The figure shows three views and two pictorial views of one solid part (mm, origin at its lowest corner). Answer the questions. Round coordinates to 2 decimals unless told otherwise and drop trailing zeros. Order: outer loops, then holes, each group sorted by start corner. A loop starts at its lowest first (then second) coordinate and runs counter-clockwise, first axis right, second up. Notation, with made-up numbers: (17, 16.25) -> (45, 16.25) arc R29 cw to (45, 39.25) -> close; hole circle Ø2 at (87, 72.25). An arc over 180 degrees is marked (long way). Return JSON: item names as keys, results as strings. Group by question number.
(1) The part is cut by section A-A (x = 67.5). Determine the outline of the cut face in (y, z), plus the area to 3 significant figures.
(2) Consider line 1 (Y direction, x = 85.5, z = 1.3); line 2 (Y direction, x = 5, z = 0.95); line 3 (X direction, y = 1, z = 1.25). Determine where each line is inside the solid, lowest interval first. Write a range as [from, to].
(3) The part is cut by section B-B (z = 1.45). Count the separate pieces of the cut face and the enclosed holes in it, plus the area to 3 significant figures.
(4) The part is cut by section C-C (y = 17). Determine the outline of the cut face in (x, z).
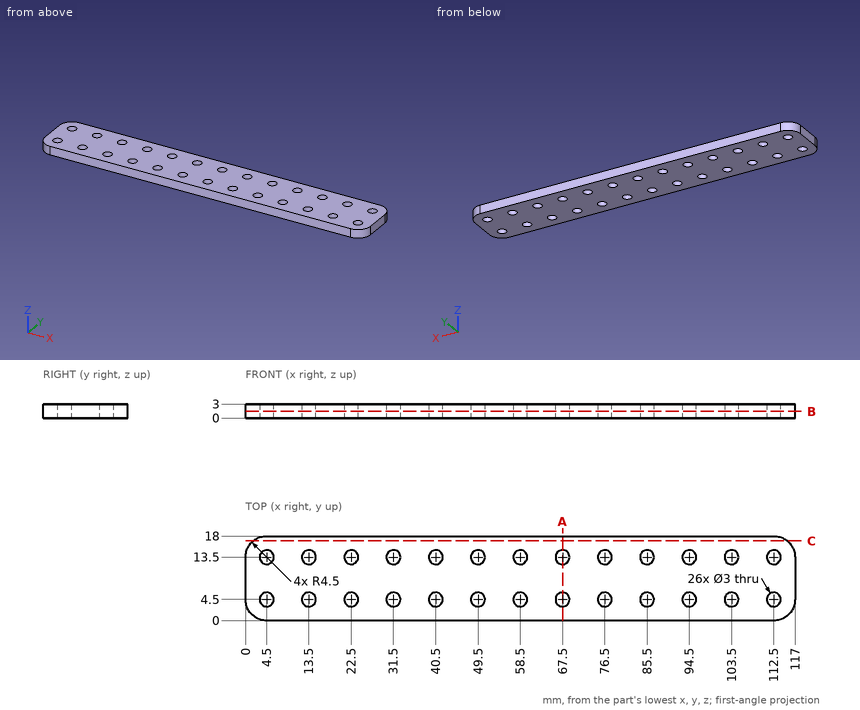
Answer below:
{
 "1": {"outline": "(0, 0) -> (3, 0) -> (3, 3) -> (0, 3) -> close; (6, 0) -> (12, 0) -> (12, 3) -> (6, 3) -> close; (15, 0) -> (18, 0) -> (18, 3) -> (15, 3) -> close", "area": "36.0 mm²"},
 "2": {"line 1": "y = [0, 3], [6, 12], [15, 18]", "line 2": "y = [0, 3.09], [5.91, 12.09], [14.91, 18]", "line 3": "x = [1.67, 115.33]"},
 "3": {"separate pieces": "1", "enclosed holes": "26", "area": "1,900 mm²"},
 "4": {"outline": "(1.67, 0) -> (115.33, 0) -> (115.33, 3) -> (1.67, 3) -> close"}
}
